```python
from build123d import *

# Parameters (mm, degrees)
F0_W     = 200
F0_H     = 100
F0_R     = 35
F1_DEPTH = 25
F3_W     = 16.588136
F3_H     = 100
F4_DEPTH = 20
F2_W     = 15
F2_H     = 103.238912
F5_DEPTH = 20


with BuildPart() as f1:
    # F0 (on Top) → F1 (new body)
    with BuildSketch(Plane.XY):
        Rectangle(F0_W, F0_H)
        Circle(F0_R, mode=Mode.SUBTRACT)
    extrude(amount=F1_DEPTH)

    # F3 (on face) → F4 (cut)
    with BuildSketch(Plane.XY.offset(25)):
        with Locations((67.693889, 0)):
            Rectangle(F3_W, F3_H)
    extrude(amount=-F4_DEPTH, mode=Mode.SUBTRACT)

    # F2 (on Top) → F5 (cut)
    with BuildSketch(Plane.XY):
        with Locations((-72.5, 0.087306)):
            Rectangle(F2_W, F2_H)
    extrude(amount=F5_DEPTH, mode=Mode.SUBTRACT)


solid = f1.part
```
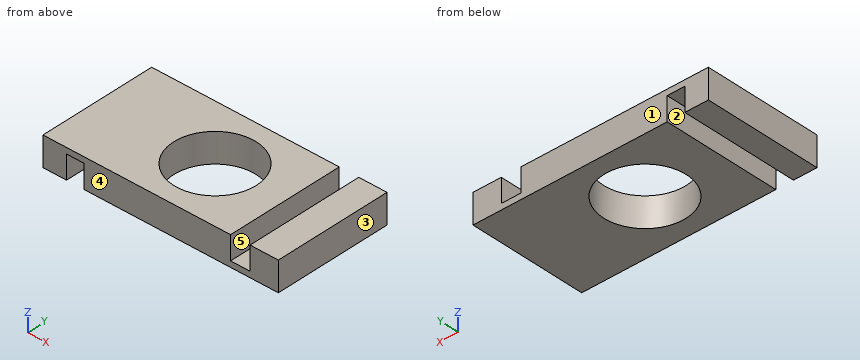
For this review, take the finished solid that the model builds, in its own axes (mm). Face numbers are marked on the shaded views. A direction names the side the tool comes from. Round coordinates to 2 decimals unless told otherwise and drop trailing zeros. Loops run counter-clockwise (first coordinate to the right, second up) from the corner with the lowest first, then second, coordinate; pieces in that order, holes last.
(1) Mouldability with a two-part tool opening along X and no side actions: class the marked faces 1, 2 and 3 as released by +X, released by -X, zero draft, split by the parting line, or undercut.
Returned:
face 1: zero draft
face 2: undercut
face 3: released by +X
(2) We need section C-C (y = 0). Give the boundary of the cut face in (x, z), plus the area to 3 significant figures.
Returned:
outline: (-100, 0) - (-80, 0) - (-80, 20) - (-65, 20) - (-65, 0) - (-35, 0) - (-35, 25) - (-100, 25) - close; (35, 0) - (100, 0) - (100, 25) - (75.99, 25) - (75.99, 5) - (59.4, 5) - (59.4, 25) - (35, 25) - close
area: 2,620 mm2
(3) We need section A-A (z = 7.75). Give the boundary of the cut face in (x, y), plus the area to 3 significant figures.
Returned:
outline: (-100, -50) - (-80, -50) - (-80, 50) - (-100, 50) - close; (-65, -50) - (59.4, -50) - (59.4, 50) - (-65, 50) - close; (75.99, -50) - (100, -50) - (100, 50) - (75.99, 50) - close; hole circle Ø70 at (0, 0)
area: 13,000 mm2
(4) We need section D-D (y = -39). Give the boundary of the cut face in (x, z), plus the area to 3 significant figures.
Returned:
outline: (-100, 0) - (-80, 0) - (-80, 20) - (-65, 20) - (-65, 0) - (100, 0) - (100, 25) - (75.99, 25) - (75.99, 5) - (59.4, 5) - (59.4, 25) - (-100, 25) - close
area: 4,370 mm2
(5) Clearance check with flat-ended pins moving along their axes: P1, Ø7.5, axis at x = -70.5, y = -18, coming from the -Z side; P2, Ø8.5, axis at x = 68, y = 21.5, coming from the +Z side. State where each tip first meets the part, or that it passes through.
Returned:
P1: stops at z = 20
P2: stops at z = 5
(6) Wall thickness on line 1 along Y through (x, z) = (0, 19.75); line 2 along X through (y, z) = (14.5, 13); line 3 along X through (y, z) = (-22.5, 1): over which ranges is each line inside the solid? List them lowest first.
Returned:
line 1: y = -50 to -35, 35 to 50
line 2: x = -100 to -80, -65 to -31.86, 31.86 to 59.4, 75.99 to 100
line 3: x = -100 to -80, -65 to -26.81, 26.81 to 100
(7) We need section B-B (x = 0). Give the boundary of the cut face in (y, z), plus the area to 3 significant figures.
Returned:
outline: (-50, 0) - (-35, 0) - (-35, 25) - (-50, 25) - close; (35, 0) - (50, 0) - (50, 25) - (35, 25) - close
area: 750 mm2
(8) Tool access review of the marked faces 4 and 5: name each direction out of +Z, -Z, +X, -X, +Y, -Y from which nothing blocks a thin tool from reaching the whole face with its end or side.
Returned:
face 4: +Z, -Z, +X, -X, -Y
face 5: +Z, +Y, -Y
